Geometry check sheet. Reference: drawing and pictorial views, mm from the part's lowest x, y, z. A direction names the side the tool comes from. Give positions to 0.01 mm unless a question says otherwise; leave off trailing zeros. Order: outer loops, then holes, each group sorted by start corner. A loop starts at its lowest first (then second) coordinate and runs counter-clockwise, first axis right, second up. Notation, with made-up numbers: (21.5, -22) - (51.5, -22) arc R22 ccw to (51.5, 17) - close; hole circle Ø11 at (66.5, -22.5). An arc over 180 degrees is marked (long way). Answer as a JSON object with one key per item and string values.
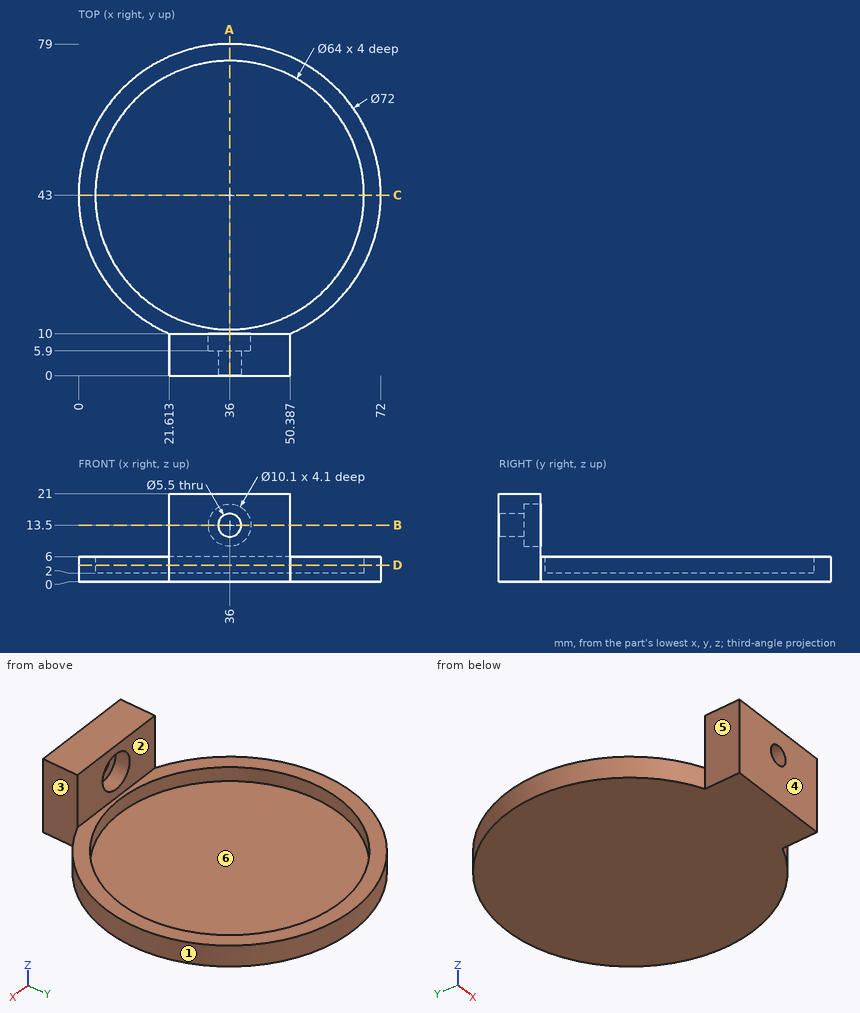
(1) Gauge pin test, flat ends, axial feed: pin 1 Ø6 at (x, y) = (33, 56.5) entering from +Z; pin 2 Ø10 at (y, z) = (15, 2.5) entering from -X (1 decimal); pin 3 Ø12 at (y, z) = (29, 10.5) entering from +X (1 decimal); pin 4 Ø3 at (x, z) = (35.5, 14) entering from +Y. Record the tip position at first contact, or that the pin passes through.
Computed values:
{"pin 1": "stops at z = 2", "pin 2": "stops at x = 8.3", "pin 3": "stops at x = 70.6", "pin 4": "passes through"}
(2) Access from +Z, -Z, +X, -X, +Y, -Y to the whole of each face (thin tool, end or side, straight path). Record for the marked faces 1, 2 and 3.
Computed values:
{"face 1": "+Z, -Z", "face 2": "+Z, +X, -X, +Y", "face 3": "+Z, -Z, +X, -Y"}
(3) Section check D-D (z = 4). Record the cut outline in (x, y), then the cut area to 3 significant figures.
Computed values:
{"outline": "(21.61, 0) - (50.39, 0) - (50.39, 10) arc R36 ccw (long way) to (21.61, 10) - close; hole circle Ø64 at (36, 43)", "area": "1,080 mm²"}
(4) Release check for a two-part mould opening along X. For the marked faces 4, 5 and 6 record: pulls with the +X half, pulls with the -X half, needs draft (parallel to the pull), parting line crosses it, or undercut.
Computed values:
{"face 4": "needs draft", "face 5": "pulls with the -X half", "face 6": "undercut"}
(5) Section check B-B (z = 13.5). Record the cut outline in (x, y), then the cut area to 3 significant figures.
Computed values:
{"outline": "(21.61, 0) - (33.25, 0) - (33.25, 5.9) - (30.95, 5.9) - (30.95, 10) - (21.61, 10) - close; (38.75, 0) - (50.39, 0) - (50.39, 10) - (41.05, 10) - (41.05, 5.9) - (38.75, 5.9) - close", "area": "214 mm²"}
(6) Section check A-A (x = 36). Record the cut outline in (y, z), then the cut area to 3 significant figures.
Computed values:
{"outline": "(0, 0) - (79, 0) - (79, 6) - (75, 6) - (75, 2) - (11, 2) - (11, 6) - (10, 6) - (10, 8.45) - (5.9, 8.45) - (5.9, 10.75) - (0, 10.75) - close; (0, 16.25) - (5.9, 16.25) - (5.9, 18.55) - (10, 18.55) - (10, 21) - (0, 21) - close", "area": "294 mm²"}
(7) Section check C-C (y = 43). Record the cut outline in (x, z), then the cut area to 3 significant figures.
Computed values:
{"outline": "(0, 0) - (72, 0) - (72, 6) - (68, 6) - (68, 2) - (4, 2) - (4, 6) - (0, 6) - close", "area": "176 mm²"}
(8) Material ranges on line 1 along Z through (x, y) = (36, 7.7); line 2 along Z through (x, y) = (36, 3.35); line 3 along Z through (x, y) = (47, 13.5), recorded low to high. Write a range as [from, to].
Computed values:
{"line 1": "z = [0, 8.45], [18.55, 21]", "line 2": "z = [0, 10.75], [16.25, 21]", "line 3": "z = [0, 2]"}
